Input: part model. Units: mm. Frame: model coordinates. A direction names the side the tool comes from. Give positions to 0.01 mm unless a question says otherwise; leave off trailing zeros. One line per item, written item: value.
Autodesk Inventor part; units mm, degrees
ref_plane "ANBAU_XY" through (0, 3.805, 3.81) normal (1, 0, 0) x (0, 0, -1)
ref_plane "ANBAU_YZ" through (0, 3.805, 3.81) normal (0, 0, -1) x (0, 1, 0)
ref_plane "ANBAU_ZX" through (0, 3.805, 3.81) normal (0, 1, 0) x (1, 0, 0)
sketch "Sketch_1" plane through (0, 0, 0) normal (0, 0, 1) x (1, 0, 0)
  line L0 (0, 0) -> (9.3, 0)
  line L1 (9.3, 0) -> (9.3, 1.2)
  line L2 (9.3, 1.2) -> (10.2, 1.2)
  line L3 (10.2, 1.2) -> (10.2, -0.3)
  line L4 (10.2, -0.3) -> (18.85, -0.3)
  arc A0 (18.85, -0.3) -> (19.15, 0) centre (18.85, 0) ccw
  line L5 (19.15, 0) -> (19.15, 9.1)
  arc A1 (19.15, 9.1) -> (18.85, 9.4) centre (18.85, 9.1) ccw
  line L6 (18.85, 9.4) -> (17.8626, 15)
  line L7 (17.8626, 15) -> (12.6, 15)
  line L8 (12.6, 15) -> (12.6, 12.1)
  line L9 (12.6, 12.1) -> (10.2, 12.1)
  line L10 (10.2, 12.1) -> (9.83, 10.7191)
  line L11 (9.83, 10.7191) -> (9.83, 7.6)
  line L12 (9.83, 7.6) -> (3, 7.6)
  line L13 (3, 7.6) -> (3, 8.5)
  line L14 (3, 8.5) -> (1.3463, 8.5)
  line L15 (1.3463, 8.5) -> (0, 8.01)
  line L16 (0, 8.01) -> (0, 0)
extrude "Extrusion1" add sketch "Sketch_1" along normal mid plane 15.04
sketch "Sketch_2" plane through (13.8, 0, 0) normal (1, 0, 0) x (0, 0, -1)
  line L0 (3.81, 12.1) -> (3.81, 17.2)
  line L1 (3.81, 17.2) -> (6.11, 17.2)
  arc A0 (6.41, 16.9) -> (6.11, 17.2) centre (6.11, 16.9) ccw
  line L2 (6.41, 16.9) -> (6.41, 12.1)
  line L3 (6.41, 12.1) -> (3.81, 12.1)
  line L4 (3.81, 12.1) -> (3.81, 17.2)
revolve "Revolution1" add sketch "Sketch_2" angle 360 about axis through (13.8, 12.1, -3.81) along (0, -1, 0)
sketch "Sketch_3" plane through (13.8, 0, 0) normal (1, 0, 0) x (0, 0, -1)
  line L0 (-3.81, 12.1) -> (-3.81, 17.2)
  line L1 (-3.81, 17.2) -> (-1.51, 17.2)
  arc A0 (-1.21, 16.9) -> (-1.51, 17.2) centre (-1.51, 16.9) ccw
  line L2 (-1.21, 16.9) -> (-1.21, 12.1)
  line L3 (-1.21, 12.1) -> (-3.81, 12.1)
  line L4 (-3.81, 12.1) -> (-3.81, 17.2)
revolve "Revolution2" add sketch "Sketch_3" angle 360 about axis through (13.8, 12.1, 3.81) along (0, -1, 0)
sketch "Sketch_4" plane through (13.8, 0, 0) normal (1, 0, 0) x (0, 0, -1)
  line L0 (3.81, 13.355) -> (3.81, 17.2)
  line L1 (3.81, 17.2) -> (5.81, 17.2)
  line L2 (5.81, 17.2) -> (5.81, 13.355)
  line L3 (5.81, 13.355) -> (3.81, 13.355)
  line L4 (3.81, 13.355) -> (3.81, 17.2)
revolve "Revolution3" cut sketch "Sketch_4" angle 360 about axis through (13.8, 13.355, -3.81) along (0, -1, 0)
sketch "Sketch_5" plane through (13.8, 0, 0) normal (1, 0, 0) x (0, 0, -1)
  line L0 (-3.81, 13.355) -> (-3.81, 17.2)
  line L1 (-3.81, 17.2) -> (-1.81, 17.2)
  line L2 (-1.81, 17.2) -> (-1.81, 13.355)
  line L3 (-1.81, 13.355) -> (-3.81, 13.355)
  line L4 (-3.81, 13.355) -> (-3.81, 17.2)
revolve "Revolution4" cut sketch "Sketch_5" angle 360 about axis through (13.8, 13.355, 3.81) along (0, -1, 0)
sketch "Sketch_6" plane through (0, 17.2, 0) normal (0, 1, 0) x (1, 0, 0)
  line L0 (13.45, 5.6775) -> (13.45, 1.9425)
  arc A0 (13.45, 1.9425) -> (14.15, 1.9425) centre (13.8, 3.81) ccw
  line L1 (14.15, 1.9425) -> (14.15, 5.6775)
  arc A1 (14.15, 5.6775) -> (13.45, 5.6775) centre (13.8, 3.81) ccw
extrude "Extrusion2" cut sketch "Sketch_6" against normal blind 4.845
sketch "Sketch_7" plane through (0, 17.2, 0) normal (0, 1, 0) x (1, 0, 0)
  line L0 (13.45, -1.9425) -> (13.45, -5.6775)
  arc A0 (13.45, -5.6775) -> (14.15, -5.6775) centre (13.8, -3.81) ccw
  line L1 (14.15, -5.6775) -> (14.15, -1.9425)
  arc A1 (14.15, -1.9425) -> (13.45, -1.9425) centre (13.8, -3.81) ccw
extrude "Extrusion3" cut sketch "Sketch_7" against normal blind 4.845
sketch "Sketch_8" plane through (18.65, 0, 0) normal (1, 0, 0) x (0, 0, -1)
  arc A0 (-6.81, 2.2) -> (-5.81, 1.2) centre (-5.81, 2.2) ccw
  line L0 (-5.81, 1.2) -> (-1.81, 1.2)
  arc A1 (-1.81, 1.2) -> (-0.81, 2.2) centre (-1.81, 2.2) ccw
  line L1 (-0.81, 2.2) -> (-0.81, 8.4)
  arc A2 (-0.81, 8.4) -> (-1.81, 9.4) centre (-1.81, 8.4) ccw
  line L2 (-1.81, 9.4) -> (-5.81, 9.4)
  arc A3 (-5.81, 9.4) -> (-6.81, 8.4) centre (-5.81, 8.4) ccw
  line L3 (-6.81, 8.4) -> (-6.81, 2.2)
  arc A4 (-6.31, 2.2) -> (-5.81, 1.7) centre (-5.81, 2.2) ccw
  line L4 (-5.81, 1.7) -> (-1.81, 1.7)
  arc A5 (-1.81, 1.7) -> (-1.31, 2.2) centre (-1.81, 2.2) ccw
  line L5 (-1.31, 2.2) -> (-1.31, 8.4)
  arc A6 (-1.31, 8.4) -> (-1.81, 8.9) centre (-1.81, 8.4) ccw
  line L6 (-1.81, 8.9) -> (-5.81, 8.9)
  arc A7 (-5.81, 8.9) -> (-6.31, 8.4) centre (-5.81, 8.4) ccw
  line L7 (-6.31, 8.4) -> (-6.31, 2.2)
extrude "Extrusion4" add sketch "Sketch_8" along normal blind 3.3
sketch "Sketch_9" plane through (18.65, 0, 0) normal (1, 0, 0) x (0, 0, -1)
  arc A0 (0.81, 2.2) -> (1.81, 1.2) centre (1.81, 2.2) ccw
  line L0 (1.81, 1.2) -> (5.81, 1.2)
  arc A1 (5.81, 1.2) -> (6.81, 2.2) centre (5.81, 2.2) ccw
  line L1 (6.81, 2.2) -> (6.81, 8.4)
  arc A2 (6.81, 8.4) -> (5.81, 9.4) centre (5.81, 8.4) ccw
  line L2 (5.81, 9.4) -> (1.81, 9.4)
  arc A3 (1.81, 9.4) -> (0.81, 8.4) centre (1.81, 8.4) ccw
  line L3 (0.81, 8.4) -> (0.81, 2.2)
  arc A4 (1.31, 2.2) -> (1.81, 1.7) centre (1.81, 2.2) ccw
  line L4 (1.81, 1.7) -> (5.81, 1.7)
  arc A5 (5.81, 1.7) -> (6.31, 2.2) centre (5.81, 2.2) ccw
  line L5 (6.31, 2.2) -> (6.31, 8.4)
  arc A6 (6.31, 8.4) -> (5.81, 8.9) centre (5.81, 8.4) ccw
  line L6 (5.81, 8.9) -> (1.81, 8.9)
  arc A7 (1.81, 8.9) -> (1.31, 8.4) centre (1.81, 8.4) ccw
  line L7 (1.31, 8.4) -> (1.31, 2.2)
extrude "Extrusion5" add sketch "Sketch_9" along normal blind 3.3
sketch "Sketch_10" plane through (0, 0, 0) normal (1, 0, 0) x (0, 1, 0)
  line L0 (6.8, 6.82) -> (1.6, 6.82)
  line L1 (1.6, 6.82) -> (1.6, 5.8691)
  arc A0 (1.6, 5.8691) -> (1.6, 1.7509) centre (3.85, 3.81) ccw
  line L2 (1.6, 1.7509) -> (1.6, 0.4)
  line L3 (1.6, 0.4) -> (6.8, 0.4)
  line L4 (6.8, 0.4) -> (6.8, 6.82)
extrude "Extrusion6" cut sketch "Sketch_10" along normal blind 8.5
sketch "Sketch_11" plane through (0, 0, 0) normal (1, 0, 0) x (0, 1, 0)
  line L0 (6.8, -0.4) -> (1.6, -0.4)
  line L1 (1.6, -0.4) -> (1.6, -1.7509)
  arc A0 (1.6, -1.7509) -> (1.6, -5.8691) centre (3.85, -3.81) ccw
  line L2 (1.6, -5.8691) -> (1.6, -6.82)
  line L3 (1.6, -6.82) -> (6.8, -6.82)
  line L4 (6.8, -6.82) -> (6.8, -0.4)
extrude "Extrusion7" cut sketch "Sketch_11" along normal blind 8.5
sketch "Sketch_12" plane through (8.5, 0, 0) normal (1, 0, 0) x (0, 0, -1)
  line L0 (-4.31, 4.305) -> (-4.31, 3.305)
  line L1 (-4.31, 3.305) -> (-3.31, 3.305)
  line L2 (-3.31, 3.305) -> (-3.31, 4.305)
  line L3 (-3.31, 4.305) -> (-4.31, 4.305)
extrude "Extrusion8" add sketch "Sketch_12" against normal blind 6.25
sketch "Sketch_13" plane through (8.5, 0, 0) normal (1, 0, 0) x (0, 0, -1)
  line L0 (3.31, 4.305) -> (3.31, 3.305)
  line L1 (3.31, 3.305) -> (4.31, 3.305)
  line L2 (4.31, 3.305) -> (4.31, 4.305)
  line L3 (4.31, 4.305) -> (3.31, 4.305)
extrude "Extrusion9" add sketch "Sketch_13" against normal blind 6.25
sketch "Sketch_14" plane through (19.15, 0, 0) normal (1, 0, 0) x (0, 0, -1)
  line L0 (15, 6) -> (15, 3)
  circle A0 centre (-3.75, 4.5) radius 1.5
revolve "Revolution5" add sketch "Sketch_14" angle 90 about axis through (19.15, 6, -15) along (0, 1, 0)
sketch "Sketch_15" plane through (19.15, 0, 0) normal (1, 0, 0) x (0, 0, -1)
  line L0 (15, 6) -> (15, 3)
  circle A0 centre (3.75, 4.5) radius 1.5
revolve "Revolution6" add sketch "Sketch_15" angle 90 about axis through (19.15, 6, -15) along (0, 1, 0)
ref_plane "ANBAU_XY" through (0, 3.805, 3.81) normal (1, 0, 0) x (0, 0, -1)
ref_plane "ANBAU_YZ" through (0, 3.805, 3.81) normal (0, 0, -1) x (0, 1, 0)
ref_plane "ANBAU_ZX" through (0, 3.805, 3.81) normal (0, 1, 0) x (1, 0, 0)
properties part number "4021832 2GD-1RR7.62-CLP-CBL"
Item 1: Material intervals for L1, parallel to X at y = 15.8, z = -3.81; L2, parallel to Z at x = 9, y = 2; L3, parallel to X at y = 9, z = 3, sorted ascending.
Verdict:
L1: x = 11.2 to 11.8, 15.8 to 16.4
L2: z = -7.52 to 7.52
L3: x = 9.83 to 21.95
Item 2: Pin query (flat end, axial travel): P1, Ø1, axis at y = 11, z = -7.5, coming from the -X side; P2, Ø3, axis at x = 21, z = 4.5, coming from the -Y side; P3, Ø6, axis at y = 4.5, z = 0, coming from the +X side. Return the tip coordinate at first contact, or that it passes through.
Verdict:
P1: stops at x = 9.83
P2: stops at y = 1.2
P3: stops at x = 35.46
Item 3: Draft query along Y for faces 5 (the face through (20.53, 1.501, 1.095)), 6 (the face through (18.363, 12.161, -0.105)), 7 (the face through (12, 6, 7.52)), 8 (the face through (19.15, 6.05, -4.4)). Return one class per face: pulls with the +Y half, pulls with the -Y half, needs draft (parallel to the pull), parting line crosses it, or undercut.
Verdict:
face 5: pulls with the -Y half
face 6: pulls with the +Y half
face 7: needs draft
face 8: undercut
Item 4: Access query for faces 1 (the face through (4, 1.6, -1)), 2 (the face through (12.6, 14, 7)), 3 (the face through (10.2, 0, 0)), 4 (the face through (21, 1.7, 4)). Directions: +Z, -Z, +X, -X, +Y, -Y. A direction counts if a zero-diameter tool reaches every point of the face in a straight line with its end or side. Return the directions, or none.
Verdict:
face 1: -X
face 2: +Z, -X, +Y
face 3: +Z, -Z, -Y
face 4: +X
